Input: part model. Units: mm. Frame: model coordinates. Face numbers are marked on the shaded views. A direction names the side the tool comes from. Round coordinates to 2 decimals unless told otherwise and drop trailing zeros. Loops run counter-clockwise (first coordinate to the right, second up) from the corner with the lowest first, then second, coordinate; pieces in that order, holes last.
(1) Access query for the marked faces 1 and 2. Directions: +Z, -Z, +X, -X, +Y, -Y. A direction counts if a zero-diameter tool reaches every point of the face in a straight line with its end or side. Return the directions, or none.
(2) Cut plane B-B, the plane y = 0. Output: boundary loops of the cut face in (x, z) (3 decimals).
(3) Cut plane D-D, the plane y = -2. Output: boundary loops of the cut face in (x, z), and give its area (3 significant figures).
(4) First-contact query: pin 1 Ø5 at (x, y) = (1.5, -4) entering from +Z; pin 2 Ø2 at (y, z) = (3, 17) entering from +X; pin 3 Ø2 at (y, z) = (2, 17) entering from +X. Flat tips, straight axial feed; report the tip coordinate or a pass-through.
(5) Cut plane A-A, the plane x = 0. Output: boundary loops of the cut face in (y, z) (3 decimals).
(6) Cut plane C-C, the plane z = 33.5. Output: boundary loops of the cut face in (x, y), and give its area (3 significant figures).
(7) Line query: line 1 (Z direction, x = -4.5, y = 3); line 2 (Z direction, x = 0.25, y = 2.25); line 3 (X direction, y = -0.75, z = 17). Output: solid intervals per line, ascending.
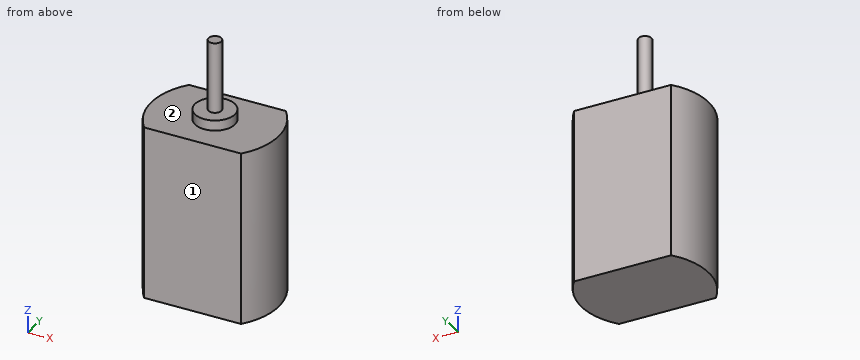
from build123d import *

# Parameters (mm, degrees)
SKETCH1_W           = 15
SKETCH1_H           = 13
BOSS_EXTRUDE1_DEPTH = 27
SKETCH2_R           = 3.075
BOSS_EXTRUDE2_DEPTH = 1.6
SKETCH3_R           = 1
BOSS_EXTRUDE3_DEPTH = 11


with BuildPart() as part:
    # Sketch1 → Boss-Extrude1 (new body)
    with BuildSketch(Plane.XY):
        Rectangle(SKETCH1_W, SKETCH1_H)
        with BuildLine():
            ThreePointArc((7.5, 6.5), (9.83933845, 0), (7.5, -6.5))
            Line((7.5, -6.5), (7.5, 6.5))
        make_face()
        with BuildLine():
            Line((-7.5, -6.5), (-7.5, 6.5))
            ThreePointArc((-7.5, 6.5), (-9.83933845, 0), (-7.5, -6.5))
        make_face()
    extrude(amount=BOSS_EXTRUDE1_DEPTH)

    # Sketch2 → Boss-Extrude2 (add)
    with BuildSketch(Plane.XY.offset(27)):
        Circle(SKETCH2_R)
    extrude(amount=BOSS_EXTRUDE2_DEPTH)

    # Sketch3 → Boss-Extrude3 (add)
    with BuildSketch(Plane.XY.offset(28.6)):
        Circle(SKETCH3_R)
    extrude(amount=BOSS_EXTRUDE3_DEPTH)


solid = part.part
Reported:
1. face 1: +Z, -Z, +X, -X, -Y
1. face 2: +Z
2. outline: (-9.839, 0) - (9.839, 0) - (9.839, 27) - (3.075, 27) - (3.075, 28.6) - (1, 28.6) - (1, 39.6) - (-1, 39.6) - (-1, 28.6) - (-3.075, 28.6) - (-3.075, 27) - (-9.839, 27) - close
3. outline: (-9.64, 0) - (9.64, 0) - (9.64, 27) - (2.34, 27) - (2.34, 28.6) - (-2.34, 28.6) - (-2.34, 27) - (-9.64, 27) - close
3. area: 528 mm2
4. pin 1: stops at z = 28.6
4. pin 2: stops at x = 9.64
4. pin 3: stops at x = 9.79
5. outline: (-6.5, 0) - (6.5, 0) - (6.5, 27) - (3.075, 27) - (3.075, 28.6) - (1, 28.6) - (1, 39.6) - (-1, 39.6) - (-1, 28.6) - (-3.075, 28.6) - (-3.075, 27) - (-6.5, 27) - close
6. outline: circle Ø2 at (0, 0)
6. area: 3.14 mm2
7. line 1: z = 0 to 27
7. line 2: z = 0 to 28.6
7. line 3: x = -9.81 to 9.81
